Check sheet for the modelled part. Datum: model origin and axes. Units: mm. A direction names the side the tool comes from. Coordinates: 2 decimals unless noted, no trailing zeros. Loops run counter-clockwise (first coordinate to the right, second up) from the corner with the lowest first, then second, coordinate; pieces in that order, holes last. Notation, with made-up numbers: M 36.5,52.5 L 49.5,52.5 A22 cw 49.5,69.5 Z; hole C -0.75,55 d4. An arc over 180 degrees is marked long. Answer in a Markdown table with one row per item. Add a question column.
Autodesk Inventor part; units mm, degrees
ref_plane "YZ Plane" through (0, 0, 0) normal (1, 0, 0) x (0, 1, 0)
ref_plane "XZ Plane" through (0, 0, 0) normal (0, 1, 0) x (-1, 0, 0)
ref_plane "XY Plane" through (0, 0, 0) normal (0, 0, 1) x (1, 0, 0)
sketch "Boceto1" plane through (0, 0, 0) normal (0, 1, 0) x (-1, 0, 0)
  line L0 (-53, -19) -> (-53, -28)
  line L1 (-50, -19) -> (-50, -28)
  line L2 (32.5, -28) -> (32.5, -25)
  line L3 (42.5, -28) -> (32.5, -28)
  line L4 (42.5, -25) -> (42.5, -28)
  line L5 (50, -12.5) -> (50, 12.5)
  line L6 (53, -12.5) -> (50, -12.5)
  line L7 (53, 12.5) -> (53, -12.5)
  line L8 (50, 12.5) -> (53, 12.5)
  line L9 (-53, 28) -> (-50, 28)
  line L10 (-53, 19) -> (-53, 28)
  line L11 (-50, 19) -> (-53, 19)
  line L12 (-50, 28) -> (-50, 19)
  line L13 (-50, -19) -> (-53, -19)
  line L14 (-53, -28) -> (-50, -28)
  line L15 (-19.5, 28) -> (-6.5, 28)
  line L16 (-19.5, 25) -> (-19.5, 28)
  line L17 (-6.5, 25) -> (-19.5, 25)
  line L18 (-6.5, 28) -> (-6.5, 25)
  line L19 (6.5, 28) -> (19.5, 28)
  line L20 (6.5, 25) -> (6.5, 28)
  line L21 (19.5, 25) -> (6.5, 25)
  line L22 (19.5, 28) -> (19.5, 25)
  line L23 (-6.5, -25) -> (-6.5, -28)
  line L24 (-19.5, -25) -> (-6.5, -25)
  line L25 (-19.5, -28) -> (-19.5, -25)
  line L26 (-6.5, -28) -> (-19.5, -28)
  line L27 (19.5, -25) -> (19.5, -28)
  line L28 (6.5, -25) -> (19.5, -25)
  line L29 (6.5, -28) -> (6.5, -25)
  line L30 (19.5, -28) -> (6.5, -28)
  line L31 (-42.5, 28) -> (-42.5, 25)
  line L32 (-32.5, 28) -> (-42.5, 28)
  line L33 (-32.5, 25) -> (-32.5, 28)
  line L34 (-42.5, 25) -> (-32.5, 25)
  line L35 (42.5, -28) -> (42.5, -25)
  line L36 (32.5, -28) -> (42.5, -28)
  line L37 (32.5, -25) -> (32.5, -28)
  line L38 (42.5, -25) -> (32.5, -25)
  line L39 (42.5, -25) -> (32.5, -25)
  line L40 (42.5, -28) -> (42.5, -25)
  line L41 (32.5, -28) -> (42.5, -28)
  line L42 (32.5, -25) -> (32.5, -28)
  line L43 (42.5, 25) -> (32.5, 25)
  line L44 (42.5, 28) -> (42.5, 25)
  line L45 (32.5, 28) -> (42.5, 28)
  line L46 (32.5, 25) -> (32.5, 28)
  line L47 (-56, 31) -> (-56, -31)
  line L48 (56, 31) -> (-56, 31)
  line L49 (56, -31) -> (56, 31)
  line L50 (-56, -31) -> (56, -31)
  line L51 (-32.5, -28) -> (-32.5, -25)
  line L52 (-42.5, -28) -> (-32.5, -28)
  line L53 (-42.5, -25) -> (-42.5, -28)
  line L54 (-32.5, -25) -> (-42.5, -25)
  point P0 (0, 0)
extrude "Extrusión1" add sketch "Boceto1" along normal blind 3
properties part number "Case_Base1" material "MDF Tablero de fibras de densidad media"
Q1. Cross-section at B-B (x = -39). Record the cut outline in (y, z), plus the area to 3 significant figures.
Q2. Access from +Z, -Z, +X, -X, +Y, -Y to the whole of each face (thin tool, end or side, straight path). Record for faces 1 (the face through (56, 1, 0)), 2 (the face through (-53, 1, 0)).
Q3. Mould release check, pull along Z, two halves, no side actions. Record for faces 3 (the face through (-1, 1, 31)), 4 (the face through (1, 3, 0)), 5 (the face through (51, 1, -19)): released by +Z, released by -Z, zero draft, split by the parting line, or undercut.
Q4. Thickness scan on L1, parallel to Z at x = 51, y = 2.3; L2, parallel to Z at x = 12.5, y = 2.45; L3, parallel to X at y = 0.2, z = -1. Record the ranges inside material, lowest first.
Q5. Cross-section at C-C (y = 1.1). Count the separate pieces of the cut face and the enclosed holes in it, plus the area to 3 significant figures.
Q6. Cross-section at A-A (z = -8.5). Record the cut outline in (x, y), plus the area to 3 significant figures.
Answer key:
| question | item | result |
|---|---|---|
| 1 | outline | M 0,-31 L 3,-31 L 3,-28 L 0,-28 Z; M 0,-25 L 3,-25 L 3,25 L 0,25 Z; M 0,28 L 3,28 L 3,31 L 0,31 Z |
| 1 | area | 168 mm^2 |
| 2 | face 1 | +Z, -Z, +X, +Y, -Y |
| 2 | face 2 | +Y, -Y |
| 3 | face 3 | released by +Z |
| 3 | face 4 | zero draft |
| 3 | face 5 | undercut |
| 4 | L1 | -31 to -28, -19 to 19, 28 to 31 |
| 4 | L2 | -31 to -28, -25 to 25, 28 to 31 |
| 4 | L3 | -56 to -53, -50 to 56 |
| 5 | separate pieces | 1 |
| 5 | enclosed holes | 11 |
| 5 | area | 6,540 mm^2 |
| 6 | outline | M -56,0 L -53,0 L -53,3 L -56,3 Z; M -50,0 L 56,0 L 56,3 L -50,3 Z |
| 6 | area | 327 mm^2 |
